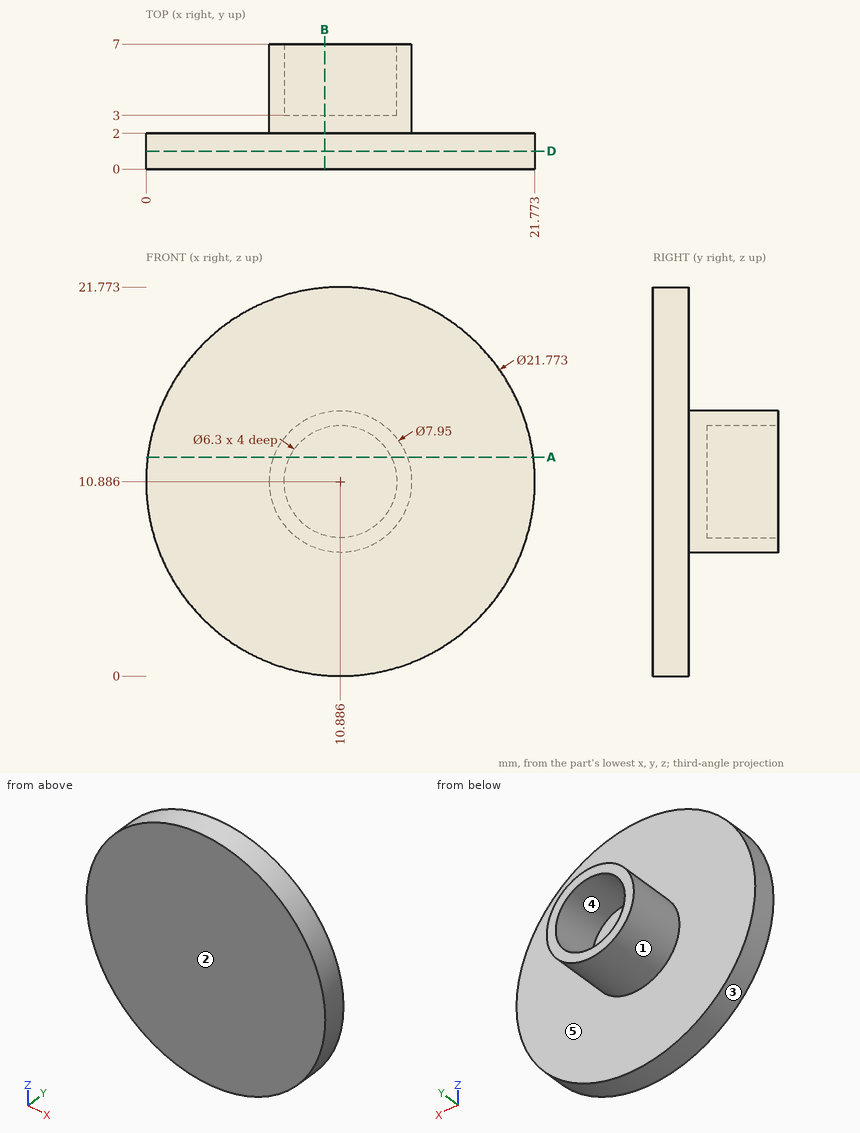
Drawing for the job (mm, zero at the part's lowest x, y, z). A direction names the side the tool comes from. Coordinates: 2 decimals unless noted, no trailing zeros. Order: outer loops, then holes, each group sorted by start corner. A loop starts at its lowest first (then second) coordinate and runs counter-clockwise, first axis right, second up.
Item 1: Drill centre lines: L1, parallel to Z at x = 11, y = 5.25 (1 decimal); L2, parallel to Y at x = 8, z = 19.5; L3, parallel to Y at x = 9.25, z = 13. Where is each one in solid material? Low to high.
Check sheet entries:
L1: z = 6.9 to 7.7, 14 to 14.9
L2: y = 0 to 2
L3: y = 0 to 3
Item 2: Band-saw the part on D-D on y = 1. List the corners of the cut face in (x, z).
Check sheet entries:
outline: circle Ø21.77 at (10.89, 10.89)
Item 3: Band-saw the part on A-A on z = 12.25. List the corners of the cut face in (x, y) (1 decimal).
Check sheet entries:
outline: (0.1, 0) - (21.7, 0) - (21.7, 2) - (14.6, 2) - (14.6, 7) - (13.7, 7) - (13.7, 3) - (8, 3) - (8, 7) - (7.2, 7) - (7.2, 2) - (0.1, 2) - close
Item 4: Two-plate mould, pull along Z, no slides. Class the marked faces 3, 4 and 5: +Z half, -Z half, draft (parallel to the pull), parting line (faces both ways), or undercut.
Check sheet entries:
face 3: parting line
face 4: undercut
face 5: draft
Item 5: Pin check, flat tips, straight feed: pin 1 Ø1.5 at (x, z) = (3, 14) entering from +Y; pin 2 Ø1 at (y, z) = (5.5, 8.5) entering from +X (1 decimal); pin 3 Ø1.9 at (x, z) = (11.5, 9.5) entering from +Y. Stop position of each tip, or through.
Check sheet entries:
pin 1: stops at y = 2
pin 2: stops at x = 14.4
pin 3: stops at y = 3
Item 6: 3-axis set-ups, long thin cutter, end or side, ignore diameter. For the marked faces 1 and 2: which of +Z, -Z, +X, -X, +Y, -Y reach the whole face in a straight line?
Check sheet entries:
face 1: +Y
face 2: +Z, -Z, +X, -X, -Y
Item 7: Band-saw the part on B-B on x = 10. List the corners of the cut face in (y, z).
Check sheet entries:
outline: (0, 0.04) - (2, 0.04) - (2, 7.01) - (7, 7.01) - (7, 7.86) - (3, 7.86) - (3, 13.91) - (7, 13.91) - (7, 14.76) - (2, 14.76) - (2, 21.74) - (0, 21.74) - close
